```python
from build123d import *

# Parameters (mm, degrees)
F1_DEPTH = 9
F3_DEPTH = 9
F4_W     = 3
F4_H     = 2
F5_DEPTH = 9.001
F6_W     = 3
F6_H     = 2
F7_DEPTH = 9.001


with BuildPart() as f1:
    # F0 (on Front) → F1 (new body)
    with BuildSketch(Plane.XZ):
        Polygon((3, 9), (0, 9), (0, 0), (10, 0), (3, 3), align=None)
    extrude(amount=-F1_DEPTH)

    # F2 (on face) → F3 (join)
    with BuildSketch(Plane.XY.offset(9)):
        Polygon((0, 9), (0, 0), (3, 0), (3, 6), (3, 9), align=None)
        Polygon((3, 9), (3, 6), (10, 9), align=None)
    extrude(amount=-F3_DEPTH)

    # F4 (on face) → F5 (cut, through all)
    with BuildSketch(Plane(origin=(0, 9, 0), x_dir=(-1, 0, 0), z_dir=(0, 1, 0))):
        with Locations((-6.5, 6)):
            Rectangle(F4_W, F4_H)
    extrude(amount=-F5_DEPTH, mode=Mode.SUBTRACT)

    # F6 (on face) → F7 (cut, through all)
    with BuildSketch(Plane(origin=(0, 0, 0), x_dir=(1, 0, 0), z_dir=(0, 0, -1))):
        with Locations((6.5, -3)):
            Rectangle(F6_W, F6_H)
    extrude(amount=-F7_DEPTH, mode=Mode.SUBTRACT)


solid = f1.part
```
Here's how the part is built. I have some questions about the finished solid (model axes, mm). A direction names the side the tool comes from. Give positions to 0.01 mm unless a question says otherwise; leave off trailing zeros. Write each loop counter-clockwise with the first axis right and the second up, starting at its lowest first coordinate (ties: lowest second). Pieces come first, ordered by that corner, then holes.
(1) On a 3-axis mill with a long thin cutter (end or side, diameter ignored), from which of +Z, -Z, +X, -X, +Y, -Y can I reach the whole of each face in a straight line? I mean faces 4 (the face through (6.5, 4.4, 1.5)), 5 (the face through (2.8, 5.4, 9)), 6 (the face through (8, 8.6, 6)), 7 (the face through (2.7, 0, 3.6)), 8 (the face through (6, 2, 1)). Say none if no direction works.
Output values:
face 4: +Z, +X, -Y
face 5: +Z, +X, -X, +Y, -Y
face 6: +Y, -Y
face 7: +Z, -Z, +X, -X, -Y
face 8: +Z, -Z
(2) Imagine slicing it at C-C, the plane x = 6.75. Write out the boundary of the cut face in (y, z), and give its area (3 significant figures).
Output values:
outline: (0, 0) - (2, 0) - (2, 1.39) - (0, 1.39) - close; (4, 0) - (9, 0) - (9, 5) - (7.61, 5) - (7.61, 1.39) - (4, 1.39) - close; (7.61, 7) - (9, 7) - (9, 9) - (7.61, 9) - close
area: 17.6 mm2
(3) Will these pins go through, and if not, where does the flat tip stop? pin 1 (1.7 mm diameter, centred on x = 6.5, y = 7.5, fed in from -Z); pin 2 (2 mm diameter, centred on y = 7.5, z = 5.5, fed in from +X); pin 3 (3 mm diameter, centred on x = 6.5, y = 5.5, fed in from +Z); pin 4 (3 mm diameter, centred on y = 2, z = 5, fed in from +X).
Output values:
pin 1: stops at z = 0
pin 2: stops at x = 8.83
pin 3: stops at z = 2.14
pin 4: stops at x = 3
(4) If I drill on L1, parallel to Z at x = 6.75, y = 8; L2, parallel to X at y = 2.5, z = 8; L3, parallel to Z at x = 5, y = 6.5, over which ranges is the centre line in solid material (lowest first)?
Output values:
L1: z = 0 to 5, 7 to 9
L2: x = 0 to 3
L3: z = 0 to 2.14
(5) Imagine slicing it at D-D, the plane y = 7.5. Write out the boundary of the cut face in (x, z).
Output values:
outline: (0, 0) - (10, 0) - (6.5, 1.5) - (6.5, 5) - (5, 5) - (5, 7) - (6.5, 7) - (6.5, 9) - (0, 9) - close
(6) Imagine slicing it at A-A, the plane y = 2.75. Write out the boundary of the cut face in (x, z).
Output values:
outline: (0, 0) - (5, 0) - (5, 2.14) - (3, 3) - (3, 9) - (0, 9) - close; (8, 0) - (10, 0) - (8, 0.86) - close
(7) Imagine slicing it at B-B, the plane z = 6.25. Write out the boundary of the cut face in (x, y), and give its area (3 significant figures).
Output values:
outline: (0, 0) - (3, 0) - (3, 6) - (5, 6.86) - (5, 9) - (0, 9) - close; (8, 8.14) - (10, 9) - (8, 9) - close
area: 33.0 mm2
(8) Thinking about a two-plate mould opening in Y: for faces 1 (the face through (6.5, 7.5, 4.6)), 2 (the face through (5, 8, 6)), 3 (the face through (6, 4, 1)), which applies, pulls with the +Y half, pulls with the -Y half, needs draft (parallel to the pull), parting line crosses it, or undercut?
Output values:
face 1: pulls with the -Y half
face 2: needs draft
face 3: undercut
